Check sheet for the modelled part. Datum: model origin and axes. Units: mm. A direction names the side the tool comes from. Round coordinates to 2 decimals unless told otherwise and drop trailing zeros. Write each loop counter-clockwise with the first axis right and the second up, starting at its lowest first coordinate (ties: lowest second). Pieces come first, ordered by that corner, then holes. Notation, with made-up numbers: (20, -37) -> (28, -37) arc R38 cw to (28, 1) -> close; hole circle Ø1 at (-23.75, 34). An arc over 180 degrees is marked (long way). Use one line per item in the form item = value. Start each with the question number.
```python
from build123d import *

# Parameters (mm, degrees)
F0_W     = 37.5
F0_H     = 26.8
F1_DEPTH = 1
F2_W     = 5
F2_H     = 7
F3_DEPTH = 3
F4_W     = 20
F4_H     = 18.8
F5_DEPTH = 1
F6_W     = 14
F6_H     = 16.8
F7_DEPTH = 2
F8_DEPTH = 2


with BuildPart() as f1:
    # F0 (on Top) → F1 (new body)
    with BuildSketch(Plane.XY):
        with Locations((18.75, 13.4)):
            Rectangle(F0_W, F0_H)
    extrude(amount=F1_DEPTH)

    # F2 (on face) → F3 (join)
    with BuildSketch(Plane.XY.offset(1)):
        with Locations((36, 14.3)):
            Rectangle(F2_W, F2_H)
    extrude(amount=F3_DEPTH)

    # F4 (on face) → F5 (join)
    with BuildSketch(Plane.XY.offset(1)):
        with Locations((10, 13.4)):
            Rectangle(F4_W, F4_H)
    extrude(amount=F5_DEPTH)

    # F6 (on face) → F7 (join)
    with BuildSketch(Plane.XY.offset(2)):
        with Locations((12, 13.4)):
            Rectangle(F6_W, F6_H)
    extrude(amount=F7_DEPTH)

    # F6 (on face) → F8 (join)
    with BuildSketch(Plane.XY.offset(2)):
        with Locations((12, 13.4)):
            Rectangle(F6_W, F6_H)
    extrude(amount=F8_DEPTH)


solid = f1.part
```
1. Tool access check on faces 4 (the face through (9.9, 22.8, 1.5)), 5 (the face through (33.5, 14, 2)), 6 (the face through (9.9, 4, 1.5)), 7 (the face through (36, 17.8, 2)). Record the directions out of +Z, -Z, +X, -X, +Y, -Y that give a thin tool (end or side, any length) a straight path to the whole face; none if there is none.
2. Sectioned sample at B-B (x = 7). Enter the section's corners in (y, z).
3. Mould release check, pull along X, two halves, no side actions. Record for faces 1 (the face through (12, 5, 3)), 2 (the face through (37.5, 13.2, 0.5)), 3 (the face through (20, 13.3, 1.5)): +X half, -X half, draft (parallel to the pull), parting line (faces both ways), or undercut.
4. Depth check by flat-ended pin: pin 1 (1 mm diameter, centred on x = 19, z = 3.5, fed in from +Y); pin 2 (0.8 mm diameter, centred on y = 19.5, z = 0.5, fed in from +X); pin 3 (2 mm diameter, centred on x = 13, z = 2.5, fed in from +Y). Enter the tip coordinate at first touch or a pass-through.
5. Sectioned sample at C-C (y = 20.5). Enter the section's corners in (x, z), and give its area (3 significant figures).
6. Sectioned sample at A-A (z = 1.6). Enter the section's corners in (x, y).
7. Scan lines: probe 1 along X at (y, z) = (17.75, 1.7); probe 2 along X at (y, z) = (15.5, 2.45); probe 3 along X at (y, z) = (19.5, 0.95). Record each from-to range of solid material in increasing order.
8. Sectioned sample at D-D (z = 3.6). Enter the section's corners in (x, y).
Returned:
q1.face_4 = +Z, +X, -X, +Y
q1.face_5 = +Z, +Y, -Y
q1.face_6 = +Z, +X, -X, -Y
q1.face_7 = +Z, +X, +Y
q2.outline = (0, 0) -> (26.8, 0) -> (26.8, 1) -> (22.8, 1) -> (22.8, 2) -> (21.8, 2) -> (21.8, 4) -> (5, 4) -> (5, 2) -> (4, 2) -> (4, 1) -> (0, 1) -> close
q3.face_1 = draft
q3.face_2 = +X half
q3.face_3 = undercut
q4.pin_1 = 21.8
q4.pin_2 = 37.5
q4.pin_3 = 22.8
q5.outline = (0, 0) -> (37.5, 0) -> (37.5, 1) -> (20, 1) -> (20, 2) -> (19, 2) -> (19, 4) -> (5, 4) -> (5, 2) -> (0, 2) -> close
q5.area = 85.5 mm^2
q6.outline = (0, 4) -> (20, 4) -> (20, 22.8) -> (0, 22.8) -> close; (33.5, 10.8) -> (38.5, 10.8) -> (38.5, 17.8) -> (33.5, 17.8) -> close
q7.probe_1 = 0 to 20, 33.5 to 38.5
q7.probe_2 = 5 to 19, 33.5 to 38.5
q7.probe_3 = 0 to 37.5
q8.outline = (5, 5) -> (19, 5) -> (19, 21.8) -> (5, 21.8) -> close; (33.5, 10.8) -> (38.5, 10.8) -> (38.5, 17.8) -> (33.5, 17.8) -> close
